```python
from build123d import *

# Parameters (mm, degrees)
F1_DEPTH = 380
F3_DEPTH = 100
F4_SIZE  = 50
F5_ANGLE = -90


with BuildPart() as f1:
    # F0 (on Top) → F1 (new body)
    with BuildSketch(Plane.XY):
        Polygon((500, 866.0254037844), (-500, 866.0254037844), (-1000, 0), (-500, -866.0254037844), (500, -866.0254037844), (1000, 0), align=None)
    extrude(amount=F1_DEPTH)

    # F2 (on face) → F3 (cut)
    with BuildSketch(Plane.XY.offset(380)):
        Polygon((-826.7949192431, 0), (-413.3974596216, -716.0254037844), (413.3974596216, -716.0254037844), (826.7949192431, 0), (413.3974596216, 716.0254037844), (-413.3974596216, 716.0254037844), align=None)
    extrude(amount=-F3_DEPTH, mode=Mode.SUBTRACT)

    # F4
    f4_edges = [f1.edges().sort_by_distance(p)[0] for p in [
        (0, 866.025404, 380),
        (750, 433.012702, 380),
        (-750, 433.012702, 380),
        (750, -433.012702, 380),
        (-750, -433.012702, 380),
        (0, -866.025404, 380),
        (0, 716.025404, 380),
        (-620.096189, 358.012702, 380),
        (-620.096189, -358.012702, 380),
        (0, -716.025404, 380),
        (620.096189, -358.012702, 380),
        (620.096189, 358.012702, 380),
    ]]
    chamfer(f4_edges, length=F4_SIZE)


with BuildPart() as f1_1:
    # F5: moved
    add(f1.part.rotate(Axis((0, -866.0254037844, 0), (-1, 0, 0)), F5_ANGLE))


solid = f1_1.part
```
CAD build for the part. Positions are in the model's coordinates, mm. A direction names the side the tool comes from. Coordinates: 2 decimals unless noted, no trailing zeros. Order: outer loops, then holes, each group sorted by start corner. A loop starts at its lowest first (then second) coordinate and runs counter-clockwise, first axis right, second up.
(1) Mould opens along Z. For faces 3 (the face through (7, -1029, 1732.051)), 4 (the face through (-732.15, -1220.68, 451.4)), 5 (the face through (-6.192, -1220.675, 125.35)) say: released by +Z, released by -Z, zero draft, split by the parting line, or undercut.
Solution:
face 3: released by +Z
face 4: released by -Z
face 5: undercut
(2) Saw through at B-B, the plane y = -1120. Write the cut outline in (x, z).
Solution:
outline: (-1000, 866.03) - (-500, 0) - (500, 0) - (1000, 866.03) - (500, 1732.05) - (-500, 1732.05) - close
(3) Saw through at A-A, the plane x = 301. Write the cut outline in (y, z), and give its area (3 significant figures).
Solution:
outline: (-1246.03, 50) - (-1196.03, 0) - (-866.03, 0) - (-866.03, 1732.05) - (-1196.03, 1732.05) - (-1246.03, 1682.05) - (-1246.03, 1632.05) - (-1196.03, 1582.05) - (-1146.03, 1582.05) - (-1146.03, 150) - (-1196.03, 150) - (-1246.03, 100) - close
area: 510,000 mm2
(4) Saw through at C-C, the plane z = 467. Write the cut outline in (x, y), and give its area (3 significant figures).
Solution:
outline: (-769.62, -1196.03) - (-711.89, -1246.03) - (-654.15, -1246.03) - (-596.42, -1196.03) - (-596.42, -1146.03) - (596.42, -1146.03) - (596.42, -1196.03) - (654.15, -1246.03) - (711.89, -1246.03) - (769.62, -1196.03) - (769.62, -866.03) - (-769.62, -866.03) - close
area: 460,000 mm2
(5) Which spindle directions (+Z, -Z, +X, -X, +Y, -Y) get a long thin tool onto all of the face, cutting with end or side? Do faces 1 (the face through (-6, -1171, 150)), 2 (the face through (753.5, -1028.715, 1292.976)). Say none if no direction does.
Solution:
face 1: -Y
face 2: +Z, +X, +Y, -Y
(6) Pin check, flat tips, straight feed: pin 1 Ø12 at (y, z) = (-1193, 1482) entering from +X; pin 2 Ø4 at (y, z) = (-1139, 257) entering from +X; pin 3 Ø2 at (y, z) = (-1115.5, 1321.5) entering from +X. Stop position of each tip, or through.
Solution:
pin 1: stops at x = 647.83
pin 2: stops at x = 649.53
pin 3: stops at x = 737.61
(7) Drill centre lines: L1, parallel to Y at x = -521, z = 792; L2, parallel to Z at x = -176.5, y = -1211; L3, parallel to X at y = -1196, z = 1532.5. Where is each one in solid material? Low to high.
Solution:
L1: y = -1146.03 to -866.03
L2: z = 14.97 to 135.03, 1597.03 to 1717.08
L3: x = -615.21 to -442.01, 442.01 to 615.21
